```python
from build123d import *

# Parameters (mm, degrees)
SKETCH1_W           = 60
SKETCH1_H           = 15
BOSS_EXTRUDE1_DEPTH = 90
SKETCH1_3_R         = 8
SKETCH1_3_W         = 60
SKETCH1_3_H         = 15
BOSS_EXTRUDE2_DEPTH = 15
SKETCH2_R           = 30
BOSS_EXTRUDE3_DEPTH = 30


with BuildPart() as part:
    # Sketch1 → Boss-Extrude1 (new body)
    with BuildSketch(Plane.XY):
        with Locations((0, -27.5)):
            Rectangle(SKETCH1_W, SKETCH1_H)
    extrude(amount=BOSS_EXTRUDE1_DEPTH)

    # Sketch1_3 → Boss-Extrude2 (add)
    # profile 1 of 2: a face of its own
    with BuildSketch(Plane.XY):
        with BuildLine():
            ThreePointArc((22.03289839, 6.599347585), (0, 23), (-22.03289839, 6.599347585))
            Line((-22.03289839, 6.599347585), (-30, -20))
            Line((-30, -20), (30, -20))
            Line((30, -20), (22.03289839, 6.599347585))
        make_face()
        Circle(SKETCH1_3_R, mode=Mode.SUBTRACT)
    # profile 2 of 2: a face of its own
    with BuildSketch(Plane.XY):
        with Locations((0, -27.5)):
            Rectangle(SKETCH1_3_W, SKETCH1_3_H)
    boss_extrude2 = extrude(amount=BOSS_EXTRUDE2_DEPTH)

    # Mirror1: Boss-Extrude2 across plane
    add(boss_extrude2.mirror(Plane.XY.offset(45)))

    # Sketch2 → Boss-Extrude3 (add)
    with BuildSketch(Plane.XZ.offset(35)):
        with Locations(Location((0, 45, 0), (0, 0, 180))):
            Circle(SKETCH2_R)
        with BuildLine():
            Line((-2, 59.866068747), (-2, 65.866068747))
            Line((-2, 65.866068747), (2, 65.866068747))
            Line((2, 65.866068747), (2, 59.866068747))
            ThreePointArc((2, 59.866068747), (0, 30), (-2, 59.866068747))
        make_face(mode=Mode.SUBTRACT)
    extrude(amount=BOSS_EXTRUDE3_DEPTH)


solid = part.part
```
Source: CAD feature listing. Evaluate the final solid. Frame: model axes, mm. A direction names the side the tool comes from. Give positions to 0.01 mm unless a question says otherwise; leave off trailing zeros. Order: outer loops, then holes, each group sorted by start corner. A loop starts at its lowest first (then second) coordinate and runs counter-clockwise, first axis right, second up.
(1) Contact query for flat-ended pins moving along their axis: P1, Ø1.8, axis at y = -43, z = 64, coming from the +X side; P2, Ø22.5, axis at x = 4.5, z = 33.5, coming from the -Y side; P3, Ø6.5, axis at y = -47.5, z = 62.5, coming from the -X side; P4, Ø2, axis at x = 0.5, y = -51.5, coming from the -Z side. Output: stop coordinate, or through.
(2) Access query for faces 1 (the face through (0, -12, 0)), 2 (the face through (0.631, -49.79, 30.013)), 3 (the face through (0, -35, 77)). Directions: +Z, -Z, +X, -X, +Y, -Y. A direction counts if a zero-diameter tool reaches every point of the face in a straight line with its end or side. Return the directions, or none.
(3) Section query C-C (y = -17). Return the cut outline in (x, z), plus the area to 3 significant figures.
(4) Section query A-A (z = 11). Return the cut outline in (x, y), plus the area to 3 significant figures.
(5) Section query B-B (x = 0.5). Return the cut outline in (y, z), plus the area to 3 significant figures.
(6) Pull-direction query (Y, two-part tool) for faces 4 (the face through (6, -8, 15)), 5 (the face through (0, -35, 12)), 6 (the face through (0, -20, 45)), 7 (the face through (-1.73, -7.81, 82.6)); classes: +Y half, -Y half, draft (parallel to the pull), parting line (faces both ways), or undercut.
(7) Section query D-D (y = -50). Return the cut outline in (x, z).
(8) Material intervals for line 1 along Z through (x, y) = (-8.5, -17.5); line 2 along Y through (x, z) = (13.5, 50); line 3 along Y through (x, z) = (-27, 46.5), sorted ascending.
Outcome:
1. P1: stops at x = 23.92
1. P2: stops at y = -65
1. P3: stops at x = -26.4
1. P4: stops at z = 15
2. face 1: -Z, +X, -X, +Y, -Y
2. face 2: -Y
2. face 3: +Z, -Y
3. outline: (-29.1, 0) - (29.1, 0) - (29.1, 15) - (-29.1, 15) - close; (-29.1, 75) - (29.1, 75) - (29.1, 90) - (-29.1, 90) - close
3. area: 1,750 mm2
4. outline: (-30, -35) - (30, -35) - (30, -20) - (22.03, 6.6) arc R23 ccw to (-22.03, 6.6) - (-30, -20) - close; hole circle Ø16 at (0, 0)
4. area: 2,610 mm2
5. outline: (-65, 15) - (-35, 15) - (-35, 0) - (-7.98, 0) - (-7.98, 15) - (-20, 15) - (-20, 75) - (-7.98, 75) - (-7.98, 90) - (-35, 90) - (-35, 75) - (-65, 75) - (-65, 65.87) - (-35, 65.87) - (-35, 30.01) - (-65, 30.01) - close; (7.98, 0) - (22.99, 0) - (22.99, 15) - (7.98, 15) - close; (7.98, 75) - (22.99, 75) - (22.99, 90) - (7.98, 90) - close
5. area: 2,880 mm2
6. face 4: draft
6. face 5: -Y half
6. face 6: +Y half
6. face 7: undercut
7. outline: circle Ø60 at (0, 45); hole (-2, 59.87) arc R15 ccw (long way) to (2, 59.87) - (2, 65.87) - (-2, 65.87) - close
8. line 1: z = 0 to 15, 75 to 90
8. line 2: y = -35 to -20
8. line 3: y = -65 to -20
